The model under review builds one solid part; all positions refer to its coordinate system, in mm. Face numbers are marked on the shaded views. A direction names the side the tool comes from. Round coordinates to 2 decimals unless told otherwise and drop trailing zeros. Loops run counter-clockwise (first coordinate to the right, second up) from the corner with the lowest first, then second, coordinate; pieces in that order, holes last. Notation, with made-up numbers: M 42,15.5 L 91,15.5 A23 cw 91,36.5 Z; hole C 30,41.5 d11. An arc over 180 degrees is marked long. Answer as a JSON object with one key per item and string values. Group by question number.
Item 1: Consider section B-B (y = 21). Give the boundary of the cut face in (x, z), and give its area (3 significant figures).
Item 2: Consider section C-C (z = -3). Give the boundary of the cut face in (x, y), and give its area (3 significant figures).
Item 3: Insertion check: P1, Ø1.5, axis at x = -16, y = 23.5, coming from the +Z side; P2, Ø2, axis at x = 3.5, z = -12.5, coming from the -Y side; P3, Ø3, axis at y = 3.5, z = 12.5, coming from the -X side. Each pin has a flat end and moves straight along its axis. Give the tip position at first contact, or say it passes through.
Item 4: Consider section A-A (x = -3). Give the boundary of the cut face in (y, z), and give its area (3 significant figures).
Item 5: The part is to be moulded in two halves that separate along Z. For the marked faces 4, 5 and 6, say which applies: +Z half, -Z half, draft (parallel to the pull), parting line (faces both ways), or undercut.
Item 6: Tool access review of the marked faces 1, 2 and 3: name each direction out of +Z, -Z, +X, -X, +Y, -Y from which nothing blocks a thin tool from reaching the whole face with its end or side.
Item 7: To check wall thickness, follow line 1 (Y direction, x = 3, z = 0); line 2 (X direction, y = 22.5, z = 0); line 3 (X direction, y = -8.5, z = -7.5). State the ranges of each line that lie inside material, in increasing order.
Item 8: Consider section D-D (y = -8.5). Give the boundary of the cut face in (x, z), and give its area (3 significant figures).
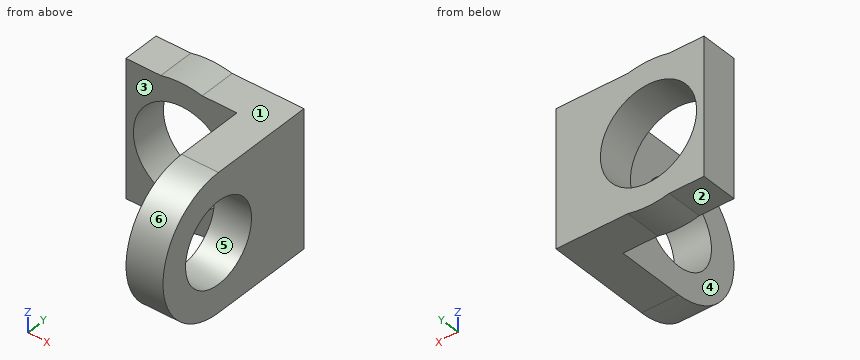
```python
from build123d import *

# Parameters (mm, degrees)
SKETCH1_R           = 18.5
SKETCH1_R_2         = 11
BOSS_EXTRUDE1_DEPTH = 10
BOSS_EXTRUDE2_REACH = 44.559
SKETCH2_W           = 10
SKETCH2_H           = 37
SKETCH2_3_R         = 13
BOSS_EXTRUDE3_DEPTH = 10


with BuildPart() as part:
    # Sketch1 → Boss-Extrude1 (new body)
    with BuildSketch(Plane(origin=(0, 0, 0), x_dir=(0, 0, -1), z_dir=(1, 0, 0))):
        Circle(SKETCH1_R)
        Circle(SKETCH1_R_2, mode=Mode.SUBTRACT)
    extrude(amount=BOSS_EXTRUDE1_DEPTH)

    # Sketch2 → Boss-Extrude2 (add, up to next)
    with BuildSketch(Plane(origin=(0, 18.5, 0), x_dir=(1, 0, 0), z_dir=(0, 1, 0)), mode=Mode.PRIVATE) as boss_extrude2_sk1:
        with Locations((5, 0)):
            Rectangle(SKETCH2_W, SKETCH2_H)
    boss_extrude2_tool1 = extrude(boss_extrude2_sk1.sketch, amount=-BOSS_EXTRUDE2_REACH, mode=Mode.PRIVATE) - part.part
    add(boss_extrude2_tool1.solids().sort_by_distance((5, 18.5, 0))[0])
    add(boss_extrude2_tool1.solids().sort_by_distance((5, 18.5, 0))[1])

    # Sketch2<3> → Boss-Extrude3 (add)
    with BuildSketch(Plane(origin=(0, 18.5, 0), x_dir=(1, 0, 0), z_dir=(0, 1, 0))):
        with BuildLine():
            Line((10, -18.5), (10, 18.5))
            Line((10, 18.5), (-9.411981237, 18.5))
            ThreePointArc((-9.411981237, 18.5), (-15, 19.153967532), (-20.588018763, 18.5))
            Line((-20.588018763, 18.5), (-30, 18.5))
            Line((-30, 18.5), (-30, -18.5))
            Line((-30, -18.5), (-20.588018763, -18.5))
            ThreePointArc((-20.588018763, -18.5), (-15, -19.153967532), (-9.411981237, -18.5))
            Line((-9.411981237, -18.5), (10, -18.5))
        make_face()
        with Locations(Location((-15, 0, 0), (0, 0, 270))):
            Circle(SKETCH2_3_R, mode=Mode.SUBTRACT)
    extrude(amount=BOSS_EXTRUDE3_DEPTH)


solid = part.part
```
Geometry results:
{
 "1": {"outline": "M -30,-18.5 L -20.59,-18.5 A24.2 ccw -9.41,-18.5 L 10,-18.5 L 10,18.5 L -9.41,18.5 A24.2 ccw -20.59,18.5 L -30,18.5 Z; hole C -15,0 d26", "area": "959 mm^2"},
 "2": {"outline": "M -30,18.5 L -27.65,18.5 L -27.65,28.5 L -30,28.5 Z; M -2.35,18.5 L 0,18.5 L 0,10.58 L 10,10.58 L 10,28.5 L -2.35,28.5 Z; M 0,-18.26 L 10,-18.26 L 10,-10.58 L 0,-10.58 Z", "area": "303 mm^2"},
 "3": {"P1": "stops at z = 19.15", "P2": "stops at y = -14.49", "P3": "stops at x = 0"},
 "4": {"outline": "M 18.5,-18.5 L 28.5,-18.5 L 28.5,-5 L 18.5,-5 Z; M 18.5,5 L 28.5,5 L 28.5,18.5 L 18.5,18.5 Z", "area": "270 mm^2"},
 "5": {"face 4": "draft", "face 5": "undercut", "face 6": "parting line"},
 "6": {"face 1": "+Z, +X, +Y, -Y", "face 2": "-Z, -X, +Y, -Y", "face 3": "+Z, -Z, -X, -Y"},
 "7": {"line 1": "y = -18.5 to -11, 11 to 28.5", "line 2": "x = -30 to -28, -2 to 10", "line 3": "x = 0 to 10"},
 "8": {"outline": "M 0,-16.43 L 10,-16.43 L 10,-6.98 L 0,-6.98 Z; M 0,6.98 L 10,6.98 L 10,16.43 L 0,16.43 Z", "area": "189 mm^2"}
}
